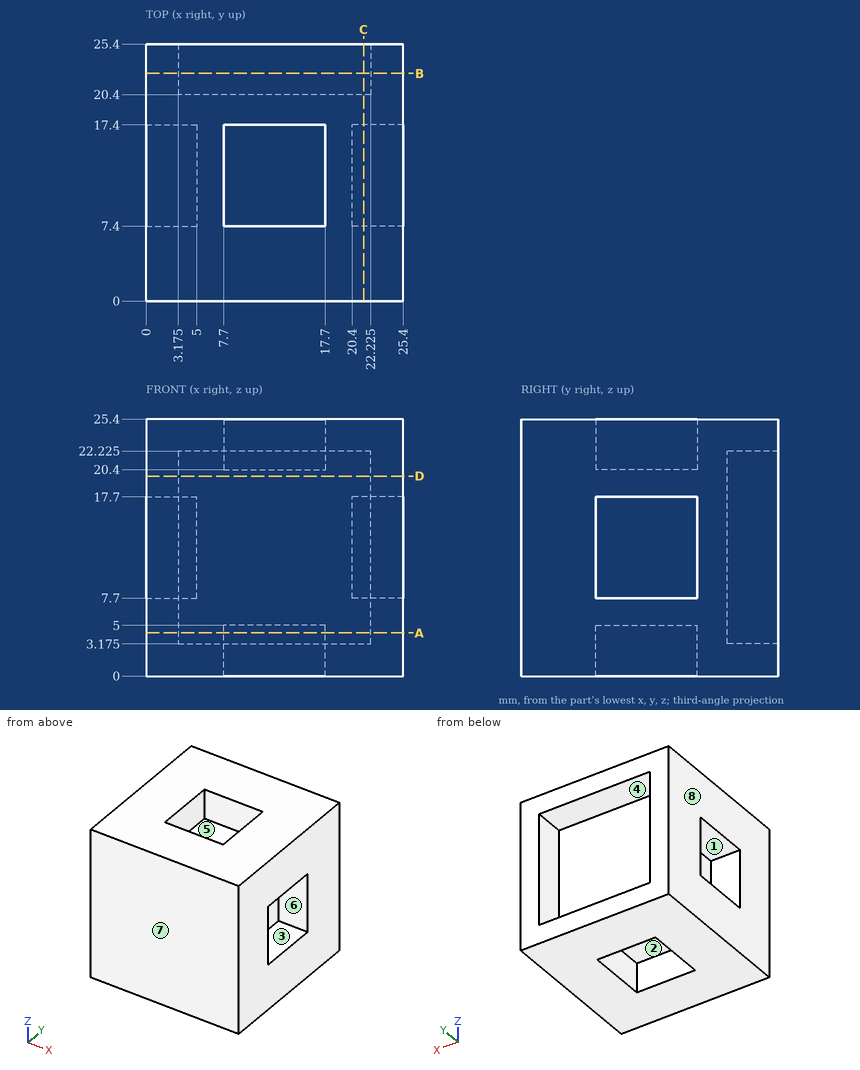
Answer from the drawing. Dimensions are ordinates in mm from the lowest x, y and z of the part. A direction names the side the tool comes from. Coordinates: 2 decimals unless noted, no trailing zeros. Order: outer loops, then holes, each group sorted by start corner. A loop starts at its lowest first (then second) coordinate and runs counter-clockwise, first axis right, second up. Notation, with made-up numbers: (-20.5, 8) - (24.5, 8) arc R25 ccw to (24.5, 44) - close; hole circle Ø6 at (81, -10). An arc over 180 degrees is marked (long way). Answer as a JSON object with one key per item and string values. Group by question number.
Item 1: Consider probe 1 along Z at (x, y) = (6.5, 22.5) (3 decimals); probe 2 along Y at (x, z) = (1.5, 11.25); probe 3 along Y at (x, z) = (15.25, 21). Determine where each line is inside the solid, lowest interval first. Write a range as from..to.
Item 2: A tool of negligible diameter and unlimited length cuts with its end or side. For the marked faces 1, 2, 3, 4 and 5, from which of +Z, -Z, +X, -X, +Y, -Y can it reach the whole face along a straight path? Write none if from no direction.
Item 3: The mould has two halves that part along Y. Classify the marked faces 6, 7 and 8: +Y half, -Y half, draft (parallel to the pull), parting line (faces both ways), or undercut.
Item 4: Flat-ended cylindrical pins translate along their axes: P1, Ø1.5, axis at x = 13.5, z = 1.5, coming from the -Y side; P2, Ø3, axis at y = 12, z = 12, coming from the -X side; P3, Ø9.5, axis at x = 12.5, z = 9.5, coming from the +Y side; P4, Ø3, axis at y = 11, z = 14.5, coming from the +X side. Find the tip coordinate at first contact, or state that the pin passes through.
Item 5: Section C-C (x = 21.5) is taken. Give the vertices of the cut face in (y, z) (3 decimals).
Item 6: Section B-B (y = 22.5) is taken. Give the vertices of the cut face in (x, z) (3 decimals).
Item 7: Section A-A (z = 4.25) is taken. Give the vertices of the cut face in (x, y) (3 decimals), plus the area to 3 significant figures.
Item 8: Section D-D (z = 19.75) is taken. Give the vertices of the cut face in (x, y) (3 decimals).
Results are:
{
 "1": {"probe 1": "z = 0..3.175, 22.225..25.4", "probe 2": "y = 0..7.4, 17.4..25.4", "probe 3": "y = 0..7.4, 17.4..20.4"},
 "2": {"face 1": "-X", "face 2": "-Z", "face 3": "+X", "face 4": "+Y", "face 5": "+Z"},
 "3": {"face 6": "undercut", "face 7": "-Y half", "face 8": "draft"},
 "4": {"P1": "stops at y = 0", "P2": "stops at x = 5", "P3": "stops at y = 20.4", "P4": "stops at x = 20.4"},
 "5": {"outline": "(0, 0) - (25.4, 0) - (25.4, 3.175) - (20.4, 3.175) - (20.4, 22.225) - (25.4, 22.225) - (25.4, 25.4) - (0, 25.4) - close; hole (7.4, 7.7) - (17.4, 7.7) - (17.4, 17.7) - (7.4, 17.7) - close"},
 "6": {"outline": "(0, 0) - (25.4, 0) - (25.4, 25.4) - (0, 25.4) - close; hole (3.175, 3.175) - (22.225, 3.175) - (22.225, 22.225) - (3.175, 22.225) - close"},
 "7": {"outline": "(0, 0) - (25.4, 0) - (25.4, 25.4) - (22.225, 25.4) - (22.225, 20.4) - (3.175, 20.4) - (3.175, 25.4) - (0, 25.4) - close; hole (7.7, 7.4) - (17.7, 7.4) - (17.7, 17.4) - (7.7, 17.4) - close", "area": "450 mm^2"},
 "8": {"outline": "(0, 0) - (25.4, 0) - (25.4, 25.4) - (22.225, 25.4) - (22.225, 20.4) - (3.175, 20.4) - (3.175, 25.4) - (0, 25.4) - close"}
}
